Could you check a few things on this drawing? It's one solid part, dimensions in mm from its lowest x, y, z. A direction names the side the tool comes from. Give positions to 0.01 mm unless a question says otherwise; leave off trailing zeros. Write each loop counter-clockwise with the first axis right and the second up, starting at its lowest first coordinate (ties: lowest second). Pieces come first, ordered by that corner, then holes. Notation, with made-up numbers: M 31,86 L 38,86 A11 ccw 38,94 Z; hole C 60.25,-22 d9. An arc over 180 degrees is marked long. Write each question's results on one line, items separated by ' | '.
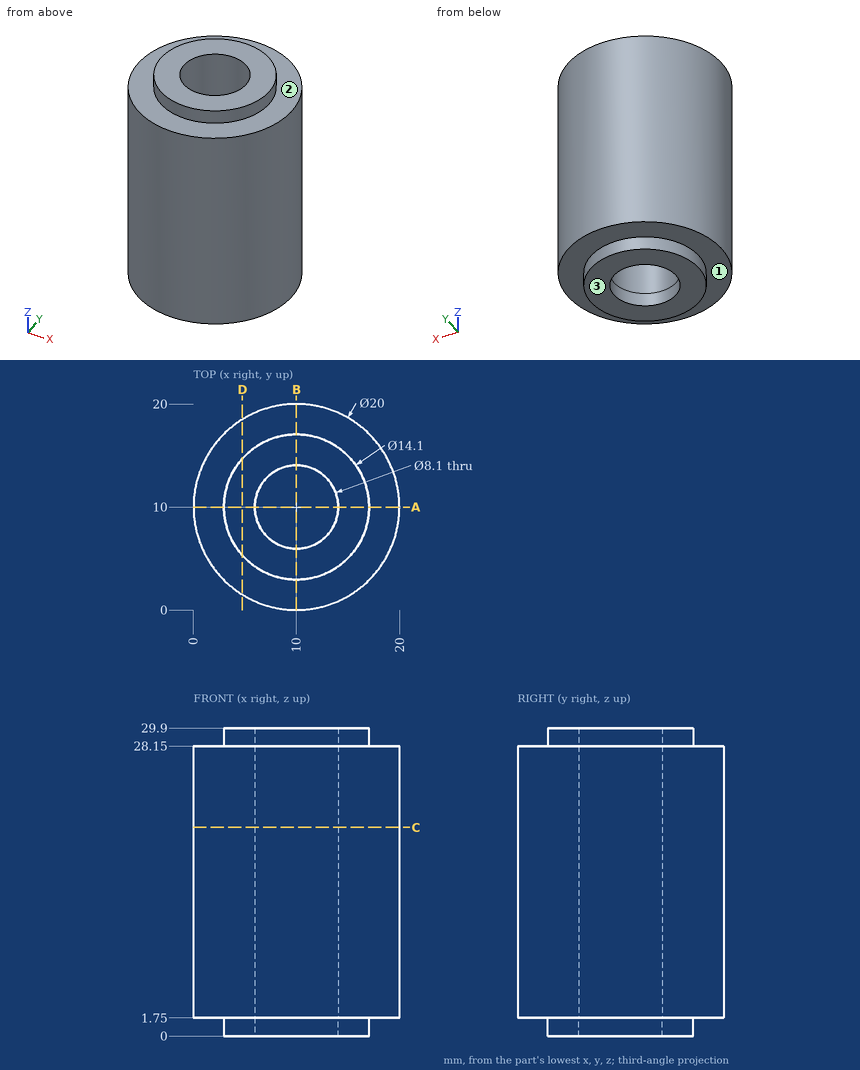
Item 1: For the marked faces 1, 2 and 3, which set-ups out of +Z, -Z, +X, -X, +Y, -Y let a thin tool reach every point of the face, with its end or its side?
Geometry says:
face 1: -Z | face 2: +Z | face 3: -Z, +X, -X, +Y, -Y
Item 2: I want a section at A-A, the plane y = 10. Please give me the cut outline in (x, z).
Geometry says:
outline: M 0,1.75 L 2.95,1.75 L 2.95,0 L 5.95,0 L 5.95,29.9 L 2.95,29.9 L 2.95,28.15 L 0,28.15 Z; M 14.05,0 L 17.05,0 L 17.05,1.75 L 20,1.75 L 20,28.15 L 17.05,28.15 L 17.05,29.9 L 14.05,29.9 Z
Item 3: I'm going to push flat-ended pins straight in: pin 1 (10 mm diameter, centred on x = 12.5, y = 11, fed in from -Z); pin 2 (1.5 mm diameter, centred on x = 2.5, y = 3, fed in from -Z); pin 3 (2 mm diameter, centred on x = 7, z = 14.5, fed in from +Y); pin 4 (1 mm diameter, centred on y = 6, z = 7.5, fed in from +X). Where does each tip first touch, or does it pass through?
Geometry says:
pin 1: stops at z = 0 | pin 2: stops at z = 1.75 | pin 3: stops at y = 19.8 | pin 4: stops at x = 19.37
Item 4: If I drill on line 1 (Y direction, x = 10, z = 1.3); line 2 (Y direction, x = 10, z = 22.5); line 3 (Z direction, x = 5.5, y = 4.5), over which ranges is the centre line in solid material (lowest first)? Write a range as from..to.
Geometry says:
line 1: y = 2.95..5.95, 14.05..17.05 | line 2: y = 0..5.95, 14.05..20 | line 3: z = 1.75..28.15
Item 5: I want a section at D-D, the plane x = 4.75. Please give me the cut outline in (y, z).
Geometry says:
outline: M 1.49,1.75 L 5.29,1.75 L 5.29,0 L 14.71,0 L 14.71,1.75 L 18.51,1.75 L 18.51,28.15 L 14.71,28.15 L 14.71,29.9 L 5.29,29.9 L 5.29,28.15 L 1.49,28.15 Z
Item 6: I want a section at C-C, the plane z = 20.25. Please give me the cut outline in (x, y), and give its area (3 significant figures).
Geometry says:
outline: C 10,10 d20; hole C 10,10 d8.1 | area: 263 mm2
